Verification items for the finished model (mm, model axes). Face numbers are marked on the shaded views. A direction names the side the tool comes from. Give positions to 0.01 mm unless a question says otherwise; leave off trailing zeros. Loops run counter-clockwise (first coordinate to the right, second up) from the corner with the lowest first, then second, coordinate; pieces in that order, holes last. Notation, with made-up numbers: M 88,20.25 L 98,20.25 A29 cw 98,50.25 Z; hole C 37,33.5 d8. An arc over 180 degrees is marked long. Use a Markdown table: item, result.
from build123d import *

# Parameters (mm, degrees)
SKETCH1_W           = 123.619311202
SKETCH1_H           = 65.206161616
BOSS_EXTRUDE1_DEPTH = 137.414
SHELL1_T            = -2.54
SKETCH2_R           = 3.216585951
SKETCH2_R_2         = 6.694232597
SKETCH2_R_3         = 10.992771438
CUT_EXTRUDE1_DEPTH  = 137.414
SKETCH3_W           = 3.463459185
SKETCH3_H           = 1.622403572
BOSS_EXTRUDE2_DEPTH = 62.666161616
SKETCH4_R           = 0.525209506
CUT_EXTRUDE2_DEPTH  = 10.668


with BuildPart() as part:
    # Sketch1 → Boss-Extrude1 (new body)
    with BuildSketch(Plane(origin=(0, 0, 0), x_dir=(1, 0, 0), z_dir=(0, 1, 0))):
        Rectangle(SKETCH1_W, SKETCH1_H)
    extrude(amount=BOSS_EXTRUDE1_DEPTH)

    # Shell1
    shell1_openings = [part.faces().sort_by_distance(p)[0] for p in [
        (0, 68.707, 32.603080808),
    ]]
    offset(amount=SHELL1_T, openings=shell1_openings, kind=Kind.INTERSECTION)

    # Sketch2 → Cut-Extrude1 (cut)
    with BuildSketch(Plane(origin=(0, 0, -32.603080808), x_dir=(-1, 0, 0), z_dir=(0, 0, -1))):
        with Locations((-42.982548284, 126.151721485)):
            Circle(SKETCH2_R)
        with Locations((-17.693943749, 108.296189209)):
            Circle(SKETCH2_R_2)
        with Locations((4.201301712, 96.419432446)):
            Circle(SKETCH2_R_3)
        with Locations(Location((4.201301712, 40.994567554, 0), (0, 0, 180))):
            Circle(SKETCH2_R_3)
        with Locations(Location((-17.693943749, 29.117810791, 0), (0, 0, 180))):
            Circle(SKETCH2_R_2)
        with Locations(Location((-42.982548284, 11.262278515, 0), (0, 0, 180))):
            Circle(SKETCH2_R)
    extrude(amount=-CUT_EXTRUDE1_DEPTH, mode=Mode.SUBTRACT)

    # Sketch3 → Boss-Extrude2 (add)
    with BuildSketch(Plane.XY.offset(-30.063080808)):
        with Locations((57.537926009, 133.950956633)):
            Rectangle(SKETCH3_W, SKETCH3_H)
        with Locations((-57.537926009, 133.950956633)):
            Rectangle(SKETCH3_W, SKETCH3_H)
        with Locations((-57.537926009, 3.463043367)):
            Rectangle(SKETCH3_W, SKETCH3_H)
        with Locations((57.537926009, 3.463043367)):
            Rectangle(SKETCH3_W, SKETCH3_H)
    extrude(amount=BOSS_EXTRUDE2_DEPTH)

    # Sketch4 → Cut-Extrude2 (cut)
    with BuildSketch(Plane.XY.offset(32.603080808)):
        with Locations((57.694217547, 133.960377278)):
            Circle(SKETCH4_R)
        with Locations(Location((-57.694217547, 133.960377278, 0), (0, 0, 180))):
            Circle(SKETCH4_R)
        with Locations(Location((57.694217547, 3.453622722, 0), (0, 0, 180))):
            Circle(SKETCH4_R)
        with Locations((-57.694217547, 3.453622722)):
            Circle(SKETCH4_R)
    extrude(amount=-CUT_EXTRUDE2_DEPTH, mode=Mode.SUBTRACT)


solid = part.part
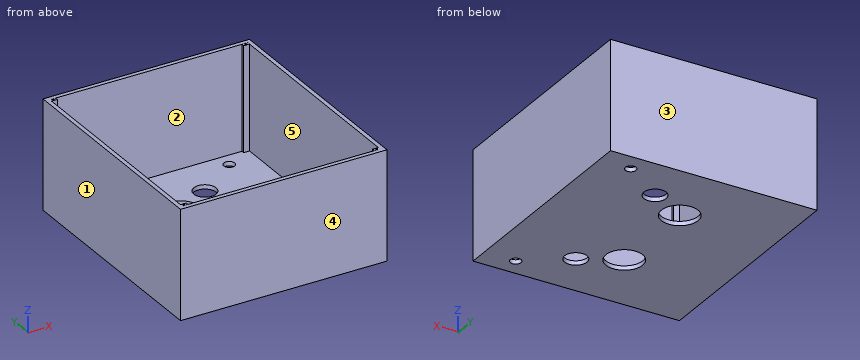
(1) Cross-section at B-B on y = 91. Record the cut outline in (x, z).
Results below:
| item | result |
|---|---|
| outline | M -61.81,-32.6 L -13.77,-32.6 L -13.77,-30.06 L -59.27,-30.06 L -59.27,32.6 L -61.81,32.6 Z; M 5.36,-32.6 L 61.81,-32.6 L 61.81,32.6 L 59.27,32.6 L 59.27,-30.06 L 5.36,-30.06 Z |
(2) Cross-section at A-A on z = -7.5. Record the cut outline in (x, y).
Results below:
| item | result |
|---|---|
| outline | M -61.81,0 L 61.81,0 L 61.81,137.41 L -61.81,137.41 Z; hole M -59.27,2.54 L 59.27,2.54 L 59.27,2.65 L 55.81,2.65 L 55.81,4.27 L 59.27,4.27 L 59.27,133.14 L 55.81,133.14 L 55.81,134.76 L 59.27,134.76 L 59.27,134.87 L -59.27,134.87 L -59.27,134.76 L -55.81,134.76 L -55.81,133.14 L -59.27,133.14 L -59.27,4.27 L -55.81,4.27 L -55.81,2.65 L -59.27,2.65 Z |
(3) Set-up check for the marked faces 4 and 5: record each of +Z, -Z, +X, -X, +Y, -Y from which the full face is reachable in a straight line by a thin tool's end or side.
Results below:
| item | result |
|---|---|
| face 4 | +Z, -Z, +X, -X, -Y |
| face 5 | +Z |
(4) Cross-section at C-C on x = 53. Record the cut outline in (y, z).
Results below:
| item | result |
|---|---|
| outline | M 0,-32.6 L 137.41,-32.6 L 137.41,32.6 L 134.87,32.6 L 134.87,-30.06 L 2.54,-30.06 L 2.54,32.6 L 0,32.6 Z |
(5) Material ranges on line 1 (Y direction, x = -44.5, z = -11.5); line 2 (X direction, y = 42.5, z = 8.5); line 3 (Z direction, x = -47.5, y = 11), recorded low to high.
Results below:
| item | result |
|---|---|
| line 1 | 0 to 2.54, 134.87 to 137.41 |
| line 2 | -61.81 to -59.27, 59.27 to 61.81 |
| line 3 | -32.6 to -30.06 |
(6) Draft check along Y on the marked faces 1, 2 and 3. Enter one of: +Y half, -Y half, draft (parallel to the pull), parting line (faces both ways), or undercut.
Results below:
| item | result |
|---|---|
| face 1 | draft |
| face 2 | undercut |
| face 3 | +Y half |
(7) Cross-section at D-D on x = -13. Record the cut outline in (y, z).
Results below:
| item | result |
|---|---|
| outline | M 0,-32.6 L 34.4,-32.6 L 34.4,-30.06 L 2.54,-30.06 L 2.54,32.6 L 0,32.6 Z; M 47.58,-32.6 L 89.83,-32.6 L 89.83,-30.06 L 47.58,-30.06 Z; M 103.01,-32.6 L 137.41,-32.6 L 137.41,32.6 L 134.87,32.6 L 134.87,-30.06 L 103.01,-30.06 Z |
(8) Gauge pin test, flat ends, axial feed: P1, Ø0.6, axis at x = -57.69, y = 133.96, coming from the +Z side; P2, Ø15.5, axis at x = 17.69, y = 108.3, coming from the +Z side. Record the tip position at first contact, or that the pin passes through.
Results below:
| item | result |
|---|---|
| P1 | z = 21.94 |
| P2 | z = -30.06 |
